```python
from build123d import *

# Parameters (mm, degrees)
F0_W     = 11.65
F0_H     = 23.75
F1_DEPTH = 20.4
F3_DEPTH = 6
F5_START = -0.8
F4_W     = 11.65
F4_H     = 4.2
F5_DEPTH = 2
F6_R     = 0.5
F7_R     = 1
F8_R     = 1.4
F9_DEPTH = 2.8
F10_R    = 4


# Not quite as in the source:
# - a feature names something its author has since deleted; it is built from what else it names


with BuildPart() as f1:
    # F0 (on Top) → F1 (new body)
    with BuildSketch(Plane.XY):
        Rectangle(F0_W, F0_H)
    extrude(amount=F1_DEPTH)

    # F2 (on face) → F3 (join)
    with BuildSketch(Plane.XY.offset(20.4)):
        with BuildLine():
            Line((5.825, 3.9640955299), (5.825, 7.5859044701))
            ThreePointArc((5.825, 7.5859044701), (0, 11.875), (-5.825, 7.5859044701))
            Line((-5.825, 7.5859044701), (-5.825, 3.9640955299))
            ThreePointArc((-5.825, 3.9640955299), (-4.7781429098, 1.9829886164), (-3.0865775367, 0.5135326087))
            ThreePointArc((-3.0865775367, 0.5135326087), (0, -3.1), (3.0865775367, 0.5135326087))
            ThreePointArc((3.0865775367, 0.5135326087), (4.7781429098, 1.9829886164), (5.825, 3.9640955299))
        make_face()
    extrude(amount=F3_DEPTH)

    # F4 (on face) → F5 (join)
    with BuildSketch(Plane.XY.offset(20.4).offset(F5_START)):
        with Locations((0, -13.975)):
            Rectangle(F4_W, F4_H)
        with Locations((0, 13.975)):
            Rectangle(F4_W, F4_H)
    extrude(amount=-F5_DEPTH)

    # F6
    f6_edges = [f1.edges().sort_by_distance(p)[0] for p in [
        (5.825, 11.875, 8.8),
        (5.825, -11.875, 8.8),
        (-5.825, -11.875, 8.8),
        (-5.825, 11.875, 8.8),
    ]]
    fillet(f6_edges, radius=F6_R)

    # F7
    f7_edges = [f1.edges().sort_by_distance(p)[0] for p in [
        (-5.825, 16.075, 18.6),
        (5.825, 16.075, 18.6),
        (5.825, -16.075, 18.6),
        (-5.825, -16.075, 18.6),
    ]]
    fillet(f7_edges, radius=F7_R)


with BuildPart() as f9:
    # F8 (on face) → F9 (new body)
    with BuildSketch(Plane.XY.offset(26.4)):
        with BuildLine():
            Line((22.5, -26), (22.5, 18.3236394078))
            Line((22.5, 18.3236394078), (1.6129450202, 18.3236394078))
            Line((1.6129450202, 18.3236394078), (-8.0251465812, 18.3236394078))
            ThreePointArc((-8.0251465812, 18.3236394078), (-10.1464669248, 17.4449597513), (-11.0251465812, 15.3236394078))
            Line((-11.0251465812, 15.3236394078), (-11.0251465812, 11.775))
            ThreePointArc((-11.0251465812, 11.775), (-11.9038262377, 9.6536796564), (-14.0251465812, 8.775))
            Line((-14.0251465812, 8.775), (-46, 8.775))
            ThreePointArc((-46, 8.775), (-49, 5.775), (-46, 2.775))
            Line((-46, 2.775), (-14.0251465812, 2.775))
            ThreePointArc((-14.0251465812, 2.775), (-11.9038262377, 1.8963203436), (-11.0251465812, -0.225))
            Line((-11.0251465812, -0.225), (-11.0251465812, -15.0673655123))
            Line((-11.0251465812, -15.0673655123), (-11.0251465812, -26))
            Line((-11.0251465812, -26), (22.5, -26))
        make_face()
        with Locations((-7.0251465812, -22)):
            Circle(F8_R, mode=Mode.SUBTRACT)
        with Locations((10.5, -22)):
            Circle(F8_R, mode=Mode.SUBTRACT)
        with Locations((-46, 5.775)):
            Circle(F8_R, mode=Mode.SUBTRACT)
        with BuildLine():
            ThreePointArc((5.825, 3.9640955299), (4.7781429098, 1.9829886164), (3.0865775367, 0.5135326087))
            ThreePointArc((3.0865775367, 0.5135326087), (0, -3.1290056936), (-3.0865775367, 0.5135326087))
            ThreePointArc((-3.0865775367, 0.5135326087), (-4.7781429098, 1.9829886164), (-5.825, 3.9640955299))
            Line((-5.825, 3.9640955299), (-5.825, 7.5859044701))
            ThreePointArc((-5.825, 7.5859044701), (0, 11.875), (5.825, 7.5859044701))
            Line((5.825, 7.5859044701), (5.825, 3.9640955299))
        make_face(mode=Mode.SUBTRACT)
        with Locations((18.5, 6)):
            Circle(F8_R, mode=Mode.SUBTRACT)
    extrude(amount=-F9_DEPTH)

    # F10
    f10_edges = [f9.edges().sort_by_distance(p)[0] for p in [
        (-11.025147, -26, 25),
        (22.5, -26, 25),
        (22.5, 18.323639, 25),
    ]]
    fillet(f10_edges, radius=F10_R)


with BuildPart() as f11_1:
    # F11: copy of F9
    add(f9.part)


solid = f9.part
```
Check sheet for the modelled part. Datum: model origin and axes. Units: mm. A direction names the side the tool comes from. Give positions to 0.01 mm unless a question says otherwise; leave off trailing zeros. Write each loop counter-clockwise with the first axis right and the second up, starting at its lowest first coordinate (ties: lowest second). Pieces come first, ordered by that corner, then holes. Notation, with made-up numbers: (86.5, 84) - (128.5, 84) arc R24 cw to (128.5, 119) - close; hole circle Ø7 at (26, 74.25). An arc over 180 degrees is marked (long way). Answer as a JSON object with one key per item and string values. Group by question number.
1) Thickness scan on probe 1 along Y at (x, z) = (18.5, 24.35); probe 2 along Y at (x, z) = (-46, 24.9) (3 decimals); probe 3 along X at (y, z) = (0, 24.6). Record the ranges inside material, lowest first. Write a range as from..to.
2) Release check for a two-part mould opening along Y. For faces 4 (the face through (-0.108, 11.874, 25.02)), 5 (the face through (-10.12, 17.47, 25.02)), 6 (the face through (-11.025, 14, 25)), 7 (the face through (-44.707, 5.239, 25.02)) record: pulls with the +Y half, pulls with the -Y half, needs draft (parallel to the pull), parting line crosses it, or undercut.
3) Sectioned sample at D-D (y = -14.5). Record the cut outline in (x, z).
4) Sectioned sample at A-A (x = 10.5). Record the cut outline in (y, z), then the cut area to 3 significant figures.
5) Sectioned sample at C-C (z = 24.5). Record the cut outline in (x, y) (3 decimals), then the cut area to 3 significant figures.
6) Sectioned sample at B-B (x = 0). Record the cut outline in (y, z) (3 decimals), then the cut area to 3 significant figures.
7) Access from +Z, -Z, +X, -X, +Y, -Y to the whole of each face (thin tool, end or side, straight path). Record for faces 1 (the face through (-30, 2.775, 25)), 2 (the face through (5.825, 6, 25)), 3 (the face through (-49, 5.8, 25)).
8) Depth check by flat-ended pin: P1, Ø2, axis at x = 10.5, y = -22, coming from the +Z side; P2, Ø1.4, axis at y = -8.5, z = 25.5, coming from the -X side; P3, Ø3.5, axis at x = -7.03, y = -22, coming from the -Z side; P4, Ø0.8, axis at y = 5, z = 25, coming from the -X side. Enter the tip coordinate at first touch or a pass-through.
Geometry results:
{
 "1": {"probe 1": "y = -26..4.6, 7.4..18.32", "probe 2": "y = 2.775..4.375, 7.175..8.775", "probe 3": "x = -11.03..-3.13, 3.13..22.5"},
 "2": {"face 4": "undercut", "face 5": "pulls with the +Y half", "face 6": "needs draft", "face 7": "undercut"},
 "3": {"outline": "(-11.03, 23.6) - (22.5, 23.6) - (22.5, 26.4) - (-11.03, 26.4) - close"},
 "4": {"outline": "(-26, 23.6) - (-23.4, 23.6) - (-23.4, 26.4) - (-26, 26.4) - close; (-20.6, 23.6) - (18.32, 23.6) - (18.32, 26.4) - (-20.6, 26.4) - close", "area": "116 mm^2"},
 "5": {"outline": "(-46, 2.775) - (-14.025, 2.775) arc R3 cw to (-11.025, -0.225) - (-11.025, -22) arc R4 ccw to (-7.025, -26) - (18.5, -26) arc R4 ccw to (22.5, -22) - (22.5, 14.324) arc R4 ccw to (18.5, 18.324) - (-8.025, 18.324) arc R3 ccw to (-11.025, 15.324) - (-11.025, 11.775) arc R3 cw to (-14.025, 8.775) - (-46, 8.775) arc R3 ccw to start; hole circle Ø2.8 at (-46, 5.775); hole circle Ø2.8 at (-7.025, -22); hole (-5.825, 3.964) arc R6.1 ccw to (-3.087, 0.514) arc R3.129 ccw (long way) to (3.087, 0.514) arc R6.1 ccw to (5.825, 3.964) - (5.825, 7.586) arc R6.1 ccw to (-5.825, 7.586) - close; hole circle Ø2.8 at (10.5, -22); hole circle Ø2.8 at (18.5, 6)", "area": "1,550 mm^2"},
 "6": {"outline": "(-26, 23.6) - (-3.129, 23.6) - (-3.129, 26.4) - (-26, 26.4) - close; (11.875, 23.6) - (18.324, 23.6) - (18.324, 26.4) - (11.875, 26.4) - close", "area": "82.1 mm^2"},
 "7": {"face 1": "+Z, -Z, -X, -Y", "face 2": "+Z, -Z", "face 3": "+Z, -Z, -X"},
 "8": {"P1": "passes through", "P2": "stops at x = -11.03", "P3": "stops at z = 23.6", "P4": "stops at x = -48.98"}
}
